Input: part model. Units: mm. Frame: model coordinates. Round coordinates to 2 decimals unless told otherwise and drop trailing zeros. Loops run counter-clockwise (first coordinate to the right, second up) from the corner with the lowest first, then second, coordinate; pieces in that order, holes last. Notation, with made-up numbers: (1, 9) -> (39, 9) arc R24 ccw to (39, 19) -> close; hole circle Ø2 at (-28.5, 16.25). An arc over 180 degrees is marked (long way). Answer as a JSON object with one key per item and string values.
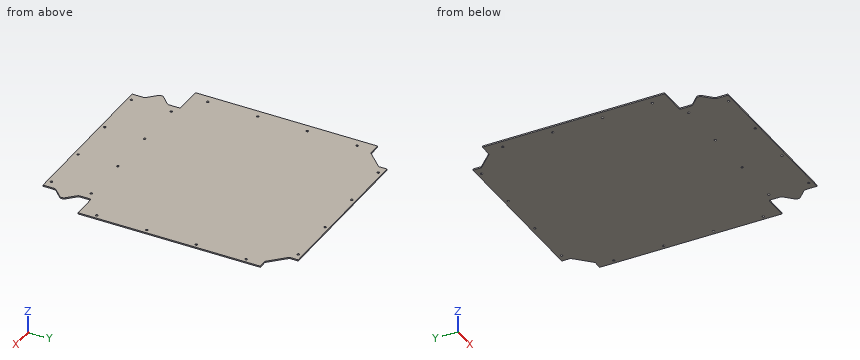
```python
from build123d import *

# Parameters (mm, degrees)
SKETCH2_W            = 550
SKETCH2_H            = 640
BOSS_EXTRUDE1_DEPTH  = 3.175
CUT_EXTRUDE1_DEPTH   = 844.866150894
FILLET1_R            = 10
FILLET2_R            = 3.175
M5_CLEARANCE_HOLE1_D = 5.8
LPATTERN1_COUNT      = 4
LPATTERN1_PITCH      = 125
M5_CLEARANCE_HOLE2_D = 5.8
LPATTERN2_COUNT      = 4
LPATTERN2_PITCH      = 125
M5_CLEARANCE_HOLE3_D = 5.8
LPATTERN3_COUNT      = 4
LPATTERN3_PITCH      = 125


with BuildPart() as part:
    # Sketch2 → Boss-Extrude1 (new body)
    with BuildSketch(Plane.XY):
        with Locations((275, 320)):
            Rectangle(SKETCH2_W, SKETCH2_H)
    extrude(amount=BOSS_EXTRUDE1_DEPTH)

    # Sketch3 → Cut-Extrude1 (cut, through all)
    with BuildSketch(Plane.XY.offset(3.175)):
        Polygon((0, 640), (0, 578), (32, 578), (72, 619), (72, 640), align=None)
        Polygon((488, 618), (488, 640), (550, 640), (550, 578), (528, 578), align=None)
        Polygon((0, 121), (71, 121), (71, 89.5), (42, 60.5), (71, 31.5), (71, 0), (0, 0), align=None)
        Polygon((550, 0), (550, 121), (488, 121), (488, 89.5), (517, 60.5), (488, 31.5), (488, 0), align=None)
    extrude(amount=-CUT_EXTRUDE1_DEPTH, mode=Mode.SUBTRACT)

    # Fillet1
    fillet1_edges = [part.edges().sort_by_distance(p)[0] for p in [
        (71, 89.5, 1.5875),
        (42, 60.5, 1.5875),
        (71, 31.5, 1.5875),
        (488, 31.5, 1.5875),
        (517, 60.5, 1.5875),
        (488, 89.5, 1.5875),
    ]]
    fillet(fillet1_edges, radius=FILLET1_R)

    # Fillet2
    fillet2_edges = [part.edges().sort_by_distance(p)[0] for p in [
        (72, 619, 1.5875),
        (32, 578, 1.5875),
        (528, 578, 1.5875),
        (488, 618, 1.5875),
        (71, 121, 1.5875),
        (488, 121, 1.5875),
    ]]
    fillet(fillet2_edges, radius=FILLET2_R)

    # M5 Clearance Hole1 (through all)
    with Locations(Plane(origin=(93.5, 630, 3.175), x_dir=(1, 0, 0), z_dir=(0, 0, 1))):
        with Locations((0, 0)):
            m5_clearance_hole1 = Hole(M5_CLEARANCE_HOLE1_D / 2)

    # LPattern1: M5 Clearance Hole1 ×4
    with Locations(*[(i * LPATTERN1_PITCH, 0, 0) for i in range(1, LPATTERN1_COUNT)]):
        add(m5_clearance_hole1, mode=Mode.SUBTRACT)

    # M5 Clearance Hole2 (through all)
    with Locations(Plane(origin=(20, 162.5, 3.175), x_dir=(1, 0, 0), z_dir=(0, 0, 1))):
        with Locations((0, 0), (520, 0)):
            m5_clearance_hole2 = Hole(M5_CLEARANCE_HOLE2_D / 2)

    # LPattern2: M5 Clearance Hole2 ×4
    with Locations(*[(0, i * LPATTERN2_PITCH, 0) for i in range(1, LPATTERN2_COUNT)]):
        add(m5_clearance_hole2, mode=Mode.SUBTRACT)

    # M5 Clearance Hole3 (through all)
    with Locations(Plane(origin=(92.5, 110, 3.175), x_dir=(1, 0, 0), z_dir=(0, 0, 1))):
        with Locations((0, 0), (0, -100)):
            m5_clearance_hole3 = Hole(M5_CLEARANCE_HOLE3_D / 2)

    # LPattern3: M5 Clearance Hole3 ×4
    with Locations(*[(i * LPATTERN3_PITCH, 0, 0) for i in range(1, LPATTERN3_COUNT)]):
        add(m5_clearance_hole3, mode=Mode.SUBTRACT)


solid = part.part
```
1) Section B-B, the plane z = 1.7. Count the separate pieces of the cut face and the enclosed holes in it, plus the area to 3 significant figures.
Output:
{"separate pieces": "1", "enclosed holes": "20", "area": "330,000 mm^2"}
2) Contact query for flat-ended pins moving along their axis: P1, Ø4.5, axis at x = 342.5, y = 10, coming from the +Z side; P2, Ø1, axis at y = 9, z = 2, coming from the -X side; P3, Ø1.6, axis at y = 103.5, z = 2, coming from the +X side; P4, Ø1, axis at x = 14, z = 1, coming from the +Y side. Output: stop coordinate, or through.
Output:
{"P1": "passes through", "P2": "stops at x = 71", "P3": "stops at x = 488", "P4": "stops at y = 578"}
3) Ray query, probe 1 along Y at (x, z) = (343.5, 1); probe 2 along Y at (x, z) = (465, 1.75); probe 3 along Y at (x, z) = (342.5, 2). Return the intervals inside material, ascending.
Output:
{"probe 1": "y = 0 to 7.28, 12.72 to 107.28, 112.72 to 627.1, 632.9 to 640", "probe 2": "y = 0 to 8.53, 11.47 to 108.53, 111.47 to 640", "probe 3": "y = 0 to 7.1, 12.9 to 107.1, 112.9 to 627.28, 632.72 to 640"}
4) Section A-A, the plane x = 60. Output: boundary loops of the cut face in (y, z) (3 decimals).
Output:
{"outline": "(42.5, 0) -> (78.5, 0) -> (78.5, 3.175) -> (42.5, 3.175) -> close; (121, 0) -> (606.7, 0) -> (606.7, 3.175) -> (121, 3.175) -> close"}
